Input: part model. Units: mm. Frame: model coordinates. A direction names the side the tool comes from. Round coordinates to 2 decimals unless told otherwise and drop trailing zeros. Loops run counter-clockwise (first coordinate to the right, second up) from the corner with the lowest first, then second, coordinate; pieces in that order, holes last. Notation, with made-up numbers: M 85,-19.75 L 103,-19.75 A22 cw 103,-9.75 Z; hole C -19.5,87 d8. An arc over 180 degrees is marked long. Put each result on its own line as item: value. Start each with the question number.
1) Section A-A on y = 6. Output: boundary loops of the cut face in (x, z).
2) Draft query along Y for faces 1 (the face through (-0.325, 16.464, 4.93)), 2 (the face through (13.14, -7.48, -0.43)), 3 (the face through (-0.26, 14.175, 4.93)), 4 (the face through (-0.1, -8.5, -1.2)). Return one class per face: +Y half, -Y half, draft (parallel to the pull), parting line (faces both ways), or undercut.
3) Section C-C on z = 3.25. Output: boundary loops of the cut face in (x, y).
4) Section B-B on x = 2.5. Output: boundary loops of the cut face in (y, z), plus the area to 3 significant figures.
5) Section D-D on x = -10. Output: boundary loops of the cut face in (y, z).
6) Reachability of faces 5 (the face through (-4, 11, -1)), 6 (the face through (4, 11, -1)), 7 (the face through (-14.181, -6.587, 4.93)) from +Z, -Z, +X, -X, +Y, -Y: full face, straight path, thin tool, end or side. Return the list, or none.
7) Pin query (flat end, axial travel): pin 1 (5 mm diameter, centred on x = 3.5, z = 0.5, fed in from -Y); pin 2 (6 mm diameter, centred on x = -1, z = -1, fed in from +Y); pin 3 (3 mm diameter, centred on y = -7.5, z = 3.5, fed in from +X); pin 4 (0.8 mm diameter, centred on y = 10.5, z = -1.5, fed in from -X). Return the tip coordinate at first contact, or that it passes through.
8) Line query: probe 1 along X at (y, z) = (-7, 3.5); probe 2 along Y at (x, z) = (0, 5.5); probe 3 along Y at (x, z) = (13, 5.25). Output: solid intervals per line, ascending.
Autodesk Inventor part; units mm, degrees
ref_plane "YZ Plane" through (0, 0, 0) normal (1, 0, 0) x (0, 1, 0)
ref_plane "XZ Plane" through (0, 0, 0) normal (0, 1, 0) x (-1, 0, 0)
ref_plane "XY Plane" through (0, 0, 0) normal (0, 0, 1) x (1, 0, 0)
sketch "Sketch3" plane through (0, 0, 0) normal (0, 0, 1) x (1, 0, 0)
  circle A0 centre (0, 0) radius 7.5
  circle A1 centre (0, 15) radius 4
  line L0 (0, 0) -> (0, 15)
  line L1 (-4, 15) -> (-4, 6.3443)
  line L2 (4, 15) -> (4, 6.3443)
  circle A2 centre (0, 0) radius 8.5
  circle A3 centre (-12.9904, -7.5) radius 4
  line L3 (-14.9904, -4.0359) -> (-7.4943, 0.292)
  line L4 (-10.9904, -10.9641) -> (-3.4943, -6.6362)
  circle A4 centre (12.9904, -7.5) radius 4
  line L5 (10.9904, -10.9641) -> (3.4943, -6.6362)
  line L6 (14.9904, -4.0359) -> (7.4943, 0.292)
  point P0 (-4, 7.5)
  point P1 (4, 7.5)
  point P2 (8.4952, -0.2859)
  point P3 (4.4952, -7.2141)
  point P4 (-4.4952, -7.2141)
  point P5 (-8.4952, -0.2859)
  dimension "d13" = 15
  dimension "d14" = 8
  dimension "d17" = 15
  dimension "d26" = 17
  dimension "d29" = 360
extrude "Extrusion3" add sketch "Sketch3" against normal blind 2.5 contours A0 L6 A2 L5 | A0 L2 A2 L6 | L5 A2 L4 A0 | A0 L0 A2 L2 | L6 A4 L5 A2 | L4 A2 L3 A0 | A0 L1 A2 L0 | A2 L0 A1 L2 | A4 | L3 A2 L1 A0 | L4 A3 L3 A2 | A2 L1 A1 L0 | A1 | A3
sketch "Sketch4" plane through (0, 0, 0) normal (0, 0, 1) x (1, 0, 0)
  arc A0 (4, 15) -> (-4, 15) centre (0, 15) ccw
  circle A1 centre (0, 15) radius 1.5
  point P0 (0, 0)
  dimension "d20" = 3
extrude "Extrusion4" add sketch "Sketch4" along normal blind 10
sketch "Sketch5" plane through (0, 0, 0) normal (0, 0, 1) x (1, 0, 0)
  circle A0 centre (0, 0) radius 7.5
  dimension "d23" = 15
pattern_circular "Circular Pattern1" count 3 over 360 about axis through (0, 0, -10) along (0, 0, 1) of "Extrusion4"
sketch "Sketch6" plane through (0, 15, 10) normal (0, 0, 1) x (1, 0, 0)
  circle A0 centre (0, 0) radius 1.5
  circle A1 centre (-12.9904, -22.5) radius 1.5
  circle A2 centre (12.9904, -22.5) radius 1.5
  point P0 (0, -15)
hole "Hole1" at (0, 15, 10) at (-12.9904, -7.5, 10) at (12.9904, -7.5, 10) direction (0, 0, -1) diameter 1.7294 depth 10 tip angle 118
properties part number "Planetery gearbox port"
Geometry results:
1. outline: M -6.02,-2.5 L -4.5,-2.5 L -4.5,0 L -6.02,0 Z; M 4.5,-2.5 L 6.02,-2.5 L 6.02,0 L 4.5,0 Z
2. face 1: parting line
2. face 2: undercut
2. face 3: undercut
2. face 4: -Y half
3. outline: C -12.99,-7.5 d3; C 0,15 d3; C 12.99,-7.5 d3; hole C -12.99,-7.5 d1.73; hole C 0,15 d1.73; hole C 12.99,-7.5 d1.73
4. outline: M -8.12,-2.5 L -7.07,-2.5 L -7.07,0 L -8.12,0 Z; M 7.07,-2.5 L 18.12,-2.5 L 18.12,0 L 7.07,0 Z
4. area: 30.3 mm²
5. outline: M -10.39,-2.5 L -1.15,-2.5 L -1.15,0 L -10.39,0 Z
6. face 5: +Z, -Z, -X, +Y
6. face 6: +Z, -Z, +X, +Y
6. face 7: +Z
7. pin 1: stops at y = -8.43
7. pin 2: stops at y = 19
7. pin 3: stops at x = 14.49
7. pin 4: stops at x = -4
8. probe 1: x = -14.4 to -13.7, -12.28 to -11.58, 11.58 to 12.28, 13.7 to 14.4
8. probe 2: y = 13.5 to 14.14, 15.86 to 16.5
8. probe 3: y = -9 to -8.36, -6.64 to -6
